Geometry: final body of the model. Coordinates: model frame, mm. Face numbers are marked on the shaded views. Coordinates: 2 decimals unless noted, no trailing zeros. Write each loop counter-clockwise with the first axis right and the second up, starting at its lowest first coordinate (ties: lowest second). Pieces come first, ordered by that corner, then holes.
from build123d import *

# Parameters (mm, degrees)
F1_W     = 127
F1_H     = 65
F1_W_2   = 122.2
F1_H_2   = 60.2
F2_DEPTH = 10
F3_DEPTH = 2.4
F4_R     = 1.5


with BuildPart() as f2:
    # F1 (on Top) → F2 (new body)
    with BuildSketch(Plane.XY):
        Rectangle(F1_W, F1_H)
        Rectangle(F1_W_2, F1_H_2, mode=Mode.SUBTRACT)
    extrude(amount=F2_DEPTH)

    # F1 (on Top) → F3 (join)
    with BuildSketch(Plane.XY):
        Rectangle(F1_W_2, F1_H_2)
    extrude(amount=F3_DEPTH)

    # F4
    f4_edges = [f2.edges().sort_by_distance(p)[0] for p in [
        (63.5, -32.5, 5),
        (63.5, 32.5, 5),
        (-63.5, 32.5, 5),
        (-63.5, -32.5, 5),
    ]]
    fillet(f4_edges, radius=F4_R)


solid = f2.part
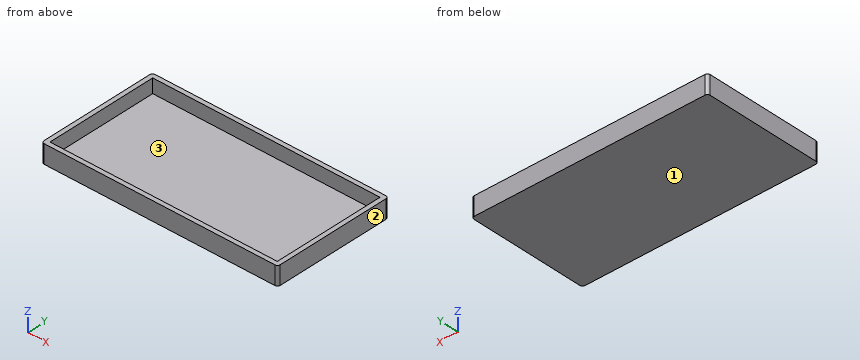
Item 1: Section B-B, the plane y = 8. Output: boundary loops of the cut face in (x, z), plus the area to 3 significant figures.
Derived:
outline: (-63.5, 0) - (63.5, 0) - (63.5, 10) - (61.1, 10) - (61.1, 2.4) - (-61.1, 2.4) - (-61.1, 10) - (-63.5, 10) - close
area: 341 mm2
Item 2: Material intervals for probe 1 along X at (y, z) = (5, 7.75); probe 2 along Y at (x, z) = (-13, 4); probe 3 along Z at (x, y) = (6, -10), sorted ascending.
Derived:
probe 1: x = -63.5 to -61.1, 61.1 to 63.5
probe 2: y = -32.5 to -30.1, 30.1 to 32.5
probe 3: z = 0 to 2.4
Item 3: Pin query (flat end, axial travel): pin 1 (10 mm diameter, centred on x = -16.5, y = 21, fed in from +Z). Return the tip coordinate at first contact, or that it passes through.
Derived:
pin 1: stops at z = 2.4
Item 4: Pull-direction query (X, two-part tool) for the marked faces 1, 2 and 3; classes: released by +X, released by -X, zero draft, split by the parting line, or undercut.
Derived:
face 1: zero draft
face 2: released by +X
face 3: undercut
Item 5: Section A-A, the plane z = 7. Output: boundary loops of the cut face in (x, y), plus the area to 3 significant figures.
Derived:
outline: (-63.5, -31) arc R1.5 ccw to (-62, -32.5) - (62, -32.5) arc R1.5 ccw to (63.5, -31) - (63.5, 31) arc R1.5 ccw to (62, 32.5) - (-62, 32.5) arc R1.5 ccw to (-63.5, 31) - close; hole (-61.1, -30.1) - (61.1, -30.1) - (61.1, 30.1) - (-61.1, 30.1) - close
area: 897 mm2
Item 6: Section C-C, the plane x = 51. Output: boundary loops of the cut face in (y, z).
Derived:
outline: (-32.5, 0) - (32.5, 0) - (32.5, 10) - (30.1, 10) - (30.1, 2.4) - (-30.1, 2.4) - (-30.1, 10) - (-32.5, 10) - close
